from build123d import *

# Parameters (mm, degrees)
SKETCH1_W           = 85
SKETCH1_H           = 60
BOSS_EXTRUDE1_DEPTH = 1
SKETCH2_W           = 65
SKETCH2_H           = 50
BOSS_EXTRUDE2_DEPTH = 6
SKETCH3_W           = 10
SKETCH3_H           = 5
BOSS_EXTRUDE3_DEPTH = 10
SKETCH4_R           = 2
CUT_EXTRUDE1_DEPTH  = 10
SKETCH5_W           = 85
SKETCH5_H           = 60
SKETCH5_R           = 2
BOSS_EXTRUDE4_DEPTH = 1
SKETCH6_R           = 3.5
SKETCH6_W           = 13
SKETCH6_H           = 12
CUT_EXTRUDE2_DEPTH  = 10
FILLET1_R           = 5
FILLET2_R           = 5
FILLET3_R           = 5
FILLET4_R           = 5


with BuildPart() as part:
    # Sketch1 → Boss-Extrude1 (new body)
    with BuildSketch(Plane(origin=(0, 0, 0), x_dir=(0, 0, -1), z_dir=(1, 0, 0))):
        with Locations((42.5, 30)):
            Rectangle(SKETCH1_W, SKETCH1_H)
    extrude(amount=BOSS_EXTRUDE1_DEPTH)

    # Sketch2 → Boss-Extrude2 (add)
    with BuildSketch(Plane(origin=(1, 0, 0), x_dir=(0, 0, -1), z_dir=(1, 0, 0))):
        with Locations((42.5, 30)):
            Rectangle(SKETCH2_W, SKETCH2_H)
    extrude(amount=BOSS_EXTRUDE2_DEPTH)

    # Sketch3 → Boss-Extrude3 (add)
    with BuildSketch(Plane(origin=(7, 0, 0), x_dir=(0, 0, -1), z_dir=(1, 0, 0))):
        with Locations((15, 7.5)):
            Rectangle(SKETCH3_W, SKETCH3_H)
        with Locations((70, 7.5)):
            Rectangle(SKETCH3_W, SKETCH3_H)
        with Locations((15, 32.5)):
            Rectangle(SKETCH3_W, SKETCH3_H)
        with Locations((70, 32.5)):
            Rectangle(SKETCH3_W, SKETCH3_H)
    extrude(amount=BOSS_EXTRUDE3_DEPTH)

    # Sketch4 → Cut-Extrude1 (cut)
    with BuildSketch(Plane(origin=(1, 0, 0), x_dir=(0, 0, -1), z_dir=(1, 0, 0))):
        with Locations((5, 30)):
            Circle(SKETCH4_R)
        with Locations((80, 30)):
            Circle(SKETCH4_R)
    extrude(amount=-CUT_EXTRUDE1_DEPTH, mode=Mode.SUBTRACT)

    # Sketch5 → Boss-Extrude4 (add)
    with BuildSketch(Plane.ZY):
        with Locations((-42.5, 30)):
            Rectangle(SKETCH5_W, SKETCH5_H)
        with Locations(Location((-80, 30, 0), (0, 0, 180))):
            Circle(SKETCH5_R, mode=Mode.SUBTRACT)
        with Locations(Location((-5, 30, 0), (0, 0, 180))):
            Circle(SKETCH5_R, mode=Mode.SUBTRACT)
    extrude(amount=BOSS_EXTRUDE4_DEPTH)

    # Sketch6 → Cut-Extrude2 (cut)
    with BuildSketch(Plane.ZY.offset(1)):
        with Locations((-42.5, 45)):
            Circle(SKETCH6_R)
        with Locations((-42.5, 20)):
            Circle(SKETCH6_R)
        with Locations((-28.5, 41)):
            Rectangle(SKETCH6_W, SKETCH6_H)
        with Locations((-28.5, 16)):
            Rectangle(SKETCH6_W, SKETCH6_H)
    extrude(amount=-CUT_EXTRUDE2_DEPTH, mode=Mode.SUBTRACT)

    # Fillet1
    fillet1_edges = [part.edges().sort_by_distance(p)[0] for p in [
        (0, 60, 0),
    ]]
    fillet(fillet1_edges, radius=FILLET1_R)

    # Fillet2
    fillet2_edges = [part.edges().sort_by_distance(p)[0] for p in [
        (0, 0, 0),
    ]]
    fillet(fillet2_edges, radius=FILLET2_R)

    # Fillet3
    fillet3_edges = [part.edges().sort_by_distance(p)[0] for p in [
        (0, 60, -85),
    ]]
    fillet(fillet3_edges, radius=FILLET3_R)

    # Fillet4
    fillet4_edges = [part.edges().sort_by_distance(p)[0] for p in [
        (0, 0, -85),
    ]]
    fillet(fillet4_edges, radius=FILLET4_R)


solid = part.part
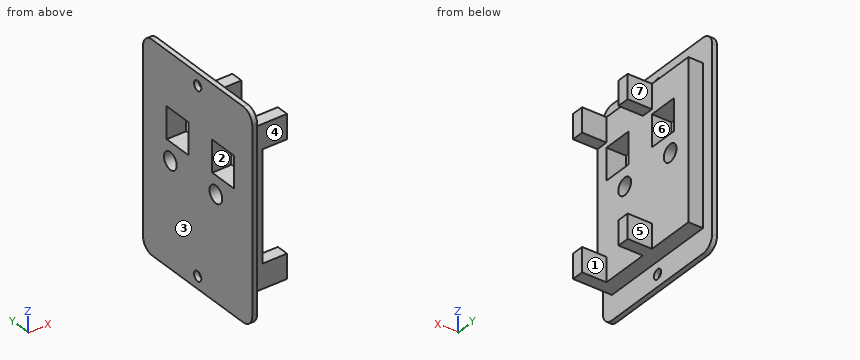
Input: part model. Units: mm. Frame: model coordinates. Face numbers are marked on the shaded views. A direction names the side the tool comes from. Coordinates: 2 decimals unless noted, no trailing zeros. Loops run counter-clockwise (first coordinate to the right, second up) from the corner with the lowest first, then second, coordinate; pieces in that order, holes last. Notation, with made-up numbers: (-18.5, 35.25) -> (35.5, 35.25) arc R22 cw to (35.5, 57.25) -> close; hole circle Ø7 at (10.25, 62.5). An arc over 180 degrees is marked (long way). Write item = value, one per line. Start each with the question number.
Item 1: Cut plane C-C, the plane x = 12.5. Return loops of the section in (y, z), plus the area to 3 significant figures.
Item 2: Material intervals for line 1 (Z direction, x = -0.2, y = 30); line 2 (Y direction, x = 2.25, z = -42.5); line 3 (Z direction, x = 15.5, y = 5.5), sorted ascending.
Item 3: Cut plane D-D, the plane y = 20. Return loops of the section in (x, z).
Item 4: Mould query, pull axis Z, two halves, no side actions, for the marked faces 6 and 7. Classes: pulls with the +Z half, pulls with the -Z half, needs draft (parallel to the pull), parting line crosses it, or undercut.
Item 5: First-contact query: P1, Ø6.5, axis at y = 20, z = -42.5, coming from the +X side; P2, Ø4, axis at x = 13.5, z = -75, coming from the +Y side; P3, Ø6, axis at x = 4.5, z = -28, coming from the +Y side; P4, Ø5, axis at x = 12.5, z = -15, coming from the -Y side. Flat tips, straight axial feed; report the tip coordinate or a pass-through.
Item 6: Cut plane B-B, the plane z = -29.5. Return loops of the section in (x, y).
Item 7: Reachability of the marked faces 1, 2, 3, 4 and 5 from +Z, -Z, +X, -X, +Y, -Y: full face, straight path, thin tool, end or side. Return the list, or none.
Item 8: Cut plane A-A, the plane y = 13.5. Return loops of the section in (x, z), plus the area to 3 significant figures.
Ans:
q1.outline = (5, -75) -> (10, -75) -> (10, -65) -> (5, -65) -> close; (5, -20) -> (10, -20) -> (10, -10) -> (5, -10) -> close; (30, -75) -> (35, -75) -> (35, -65) -> (30, -65) -> close; (30, -20) -> (35, -20) -> (35, -10) -> (30, -10) -> close
q1.area = 200 mm²
q2.line_1 = -85 to -82, -78 to -7, -3 to 0
q2.line_2 = 5 to 16.5, 23.5 to 41.5, 48.5 to 55
q2.line_3 = -75 to -65, -20 to -10
q3.outline = (-1, -85) -> (1, -85) -> (1, -75) -> (7, -75) -> (7, -46) -> (-1, -46) -> close; (-1, -39) -> (7, -39) -> (7, -35) -> (-1, -35) -> close; (-1, -22) -> (7, -22) -> (7, -10) -> (1, -10) -> (1, 0) -> (-1, 0) -> close
q4.face_6 = undercut
q4.face_7 = needs draft
q5.P1 = through
q5.P2 = 35
q5.P3 = 55
q5.P4 = 5
q6.outline = (-1, 0) -> (1, 0) -> (1, 5) -> (7, 5) -> (7, 10) -> (-1, 10) -> close; (-1, 22) -> (7, 22) -> (7, 35) -> (-1, 35) -> close; (-1, 47) -> (7, 47) -> (7, 55) -> (1, 55) -> (1, 60) -> (-1, 60) -> close
q7.face_1 = +Z, -Z, +X
q7.face_2 = +X, -X
q7.face_3 = +Z, -Z, -X, +Y, -Y
q7.face_4 = +Z, -Z, +X, -Y
q7.face_5 = +Z, -Z, +X, +Y
q8.outline = (-1, -85) -> (1, -85) -> (1, -75) -> (7, -75) -> (7, -35) -> (-1, -35) -> close; (-1, -22) -> (7, -22) -> (7, -10) -> (1, -10) -> (1, 0) -> (-1, 0) -> close
q8.area = 456 mm²
